Check sheet for the modelled part. Datum: model origin and axes. Units: mm. Face numbers are marked on the shaded views. A direction names the side the tool comes from. Coordinates: 2 decimals unless noted, no trailing zeros. Order: outer loops, then holes, each group sorted by start corner. A loop starts at its lowest first (then second) coordinate and runs counter-clockwise, first axis right, second up. Notation, with made-up numbers: M 18,6.25 L 31,6.25 A8 ccw 31,16.25 Z; hole C -24.75,78 d6. An arc over 180 degrees is marked long. Answer in a Markdown table with one row per item. Add a question column.
from build123d import *

# Parameters (mm, degrees)
SKETCH1_R           = 3.683
BOSS_EXTRUDE1_DEPTH = 63.5
SKETCH7_R           = 2.09
CUT_EXTRUDE1_DEPTH  = 20.32
SKETCH8_OUTSIDE_W   = 22.236
SKETCH8_OUTSIDE_H   = 22.236
SKETCH8_OUTSIDE_W_2 = 5.20854855
SKETCH8_OUTSIDE_H_2 = 5.20854855
CUT_EXTRUDE3_DEPTH  = 3.81


with BuildPart() as part:
    # Sketch1 → Boss-Extrude1 (new body)
    with BuildSketch(Plane(origin=(0, 0, 0), x_dir=(1, 0, 0), z_dir=(0, 1, 0))):
        Circle(SKETCH1_R)
    extrude(amount=BOSS_EXTRUDE1_DEPTH)

    # Sketch7 → Cut-Extrude1 (cut)
    with BuildSketch(Plane.XZ):
        Circle(SKETCH7_R)
    cut_extrude1 = extrude(amount=-CUT_EXTRUDE1_DEPTH, mode=Mode.SUBTRACT)

    # Mirror1: Cut-Extrude1 across plane
    add(cut_extrude1.mirror(Plane(origin=(0, 31.75, 0), x_dir=(0, 0, 1), z_dir=(0, -1, 0))), mode=Mode.SUBTRACT)

    # Sketch8 outside → Cut-Extrude3 (cut, symmetric)
    with BuildSketch(Plane(origin=(0, 31.75, 0), x_dir=(-1, 0, 0), z_dir=(0, -1, 0))):
        Rectangle(SKETCH8_OUTSIDE_W, SKETCH8_OUTSIDE_H)
        Rectangle(SKETCH8_OUTSIDE_W_2, SKETCH8_OUTSIDE_H_2, mode=Mode.SUBTRACT)
    extrude(amount=CUT_EXTRUDE3_DEPTH, both=True, mode=Mode.SUBTRACT)


solid = part.part
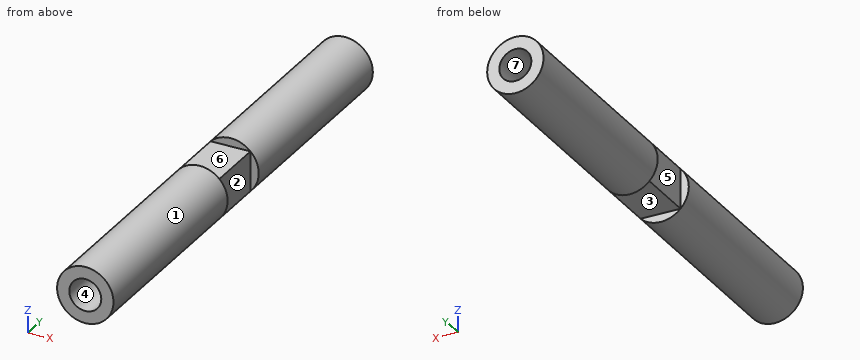
1. Section check B-B on z = 0. Enter the section's corners in (x, y).
2. Scan lines: line 1 (Y direction, x = -1.75, z = 2.75); line 2 (Z direction, x = 0, y = 55.5); line 3 (Z direction, x = -1.25, y = 50) (3 decimals). Record each from-to range of solid material in increasing order.
3. Section check D-D on y = 23.5. Enter the section's corners in (x, z).
4. Section check A-A on x = 0. Enter the section's corners in (y, z).
5. Set-up check for the marked faces 1, 2, 3 and 4: record each of +Z, -Z, +X, -X, +Y, -Y from which the full face is reachable in a straight line by a thin tool's end or side.
6. Go/stop test with flat-tipped pins: pin 1 Ø0.9 at (x, z) = (-0.5, -3) entering from -Y; pin 2 Ø2.5 at (x, z) = (0, 0) entering from +Y. Record where each tip stops, or that it passes through.
7. Release check for a two-part mould opening along X. For the marked faces 5, 6 and 7 record: released by +X, released by -X, zero draft, split by the parting line, or undercut.
8. Section check C-C on y = 14. Enter the section's corners in (x, z), then the cut area to 3 significant figures.
Result sheet:
| question | item | result |
|---|---|---|
| 1 | outline | M -3.68,0 L -2.09,0 L -2.09,20.32 L 2.09,20.32 L 2.09,0 L 3.68,0 L 3.68,27.94 L 2.6,27.94 L 2.6,35.56 L 3.68,35.56 L 3.68,63.5 L 2.09,63.5 L 2.09,43.18 L -2.09,43.18 L -2.09,63.5 L -3.68,63.5 L -3.68,35.56 L -2.6,35.56 L -2.6,27.94 L -3.68,27.94 Z |
| 2 | line 1 | 0 to 27.94, 35.56 to 63.5 |
| 2 | line 2 | -3.68 to -2.09, 2.09 to 3.68 |
| 2 | line 3 | -3.464 to -1.675, 1.675 to 3.464 |
| 3 | outline | C 0,0 d7.37 |
| 4 | outline | M 0,-3.68 L 27.94,-3.68 L 27.94,-2.6 L 35.56,-2.6 L 35.56,-3.68 L 63.5,-3.68 L 63.5,-2.09 L 43.18,-2.09 L 43.18,2.09 L 63.5,2.09 L 63.5,3.68 L 35.56,3.68 L 35.56,2.6 L 27.94,2.6 L 27.94,3.68 L 0,3.68 L 0,2.09 L 20.32,2.09 L 20.32,-2.09 L 0,-2.09 Z |
| 5 | face 1 | +Y, -Y |
| 5 | face 2 | +Z, -Z, +X |
| 5 | face 3 | -Z, +X, -X |
| 5 | face 4 | -Y |
| 6 | pin 1 | y = 0 |
| 6 | pin 2 | y = 43.18 |
| 7 | face 5 | released by -X |
| 7 | face 6 | zero draft |
| 7 | face 7 | undercut |
| 8 | outline | C 0,0 d7.37; hole C 0,0 d4.18 |
| 8 | area | 28.9 mm^2 |
